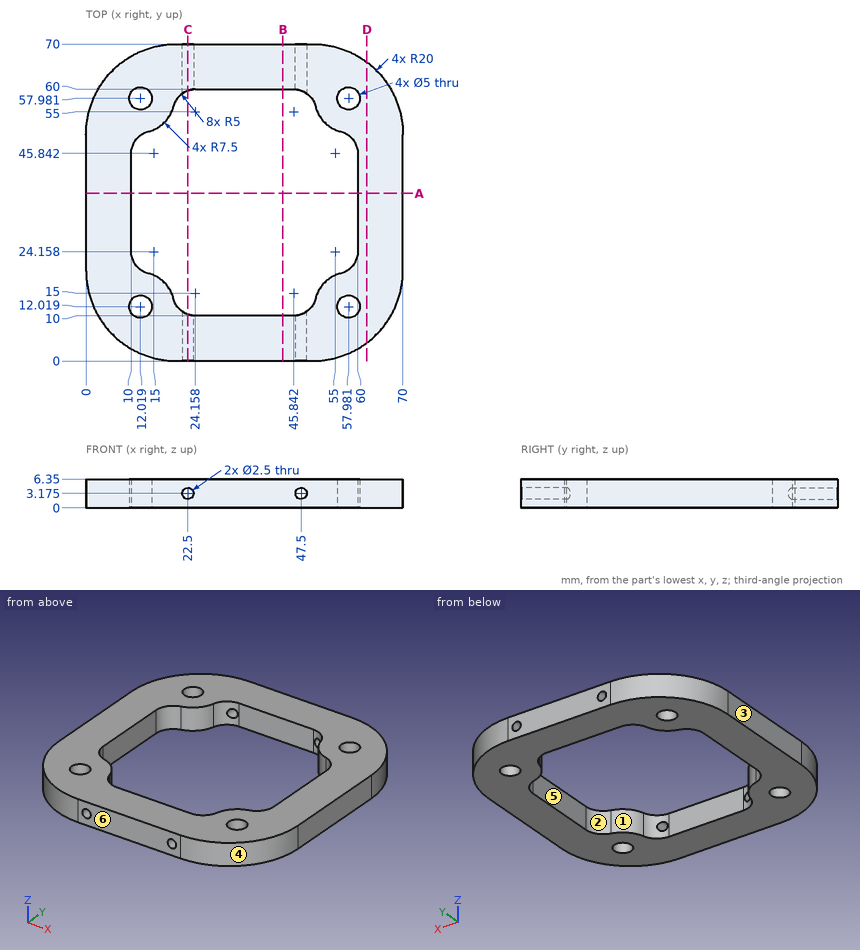
Answer from the drawing. Dimensions are ordinates in mm from the lowest x, y and z of the part. A direction names the side the tool comes from. Give positions to 0.01 mm unless a question says otherwise; leave off trailing zeros. Write each loop counter-clockwise with the first axis right and the second up, starting at its lowest first coordinate (ties: lowest second). Pieces come first, ordered by that corner, then holes. Notation, with made-up numbers: (-28, 40) - (16, 40) arc R32 cw to (16, 73) - close; hole circle Ø9 at (34, 36). An arc over 180 degrees is marked (long way). Answer in a Markdown table with one row per item. Add a question column.
Item 1: A tool of negligible diameter and unlimited length cuts with its end or side. For the marked faces 5 and 6, from which of +Z, -Z, +X, -X, +Y, -Y can it reach the whole face along a straight path? Write none if from no direction.
Item 2: Section A-A, the plane y = 37 is taken. Write down the section's boundary in (x, z), and give its area (3 significant figures).
Item 3: Determine the mould class of the marked faces 1, 2, 3 and 4 for opening direction Y: pulls with the +Y half, pulls with the -Y half, needs draft (parallel to the pull), parting line crosses it, or undercut.
Item 4: Flat-ended cylindrical pins translate along their axes: P1, Ø3, axis at y = 10, z = 5.5, coming from the -X side; P2, Ø1, axis at y = 56.5, z = 2.5, coming from the +X side. Find the tip coordinate at first contact, or state that the pin passes through.
Item 5: Section D-D, the plane x = 62 is taken. Write down the section's boundary in (y, z).
Item 6: Find the intervals of material crossed by L1, parallel to X at y = 28.5, z = 2.25; L2, parallel to Y at x = 10.5, z = 3 (1 decimal), in increasing order.
Item 7: Section C-C, the plane x = 22.5 is taken. Count the separate pieces of the cut face and the enclosed holes in it.
Recorded:
| question | item | result |
|---|---|---|
| 1 | face 5 | +Z, -Z |
| 1 | face 6 | +Z, -Z, +X, -X, -Y |
| 2 | outline | (0, 0) - (10, 0) - (10, 6.35) - (0, 6.35) - close; (60, 0) - (70, 0) - (70, 6.35) - (60, 6.35) - close |
| 2 | area | 127 mm2 |
| 3 | face 1 | undercut |
| 3 | face 2 | undercut |
| 3 | face 3 | needs draft |
| 3 | face 4 | pulls with the -Y half |
| 4 | P1 | stops at x = 1.9 |
| 4 | P2 | stops at x = 69.08 |
| 5 | outline | (4, 0) - (66, 0) - (66, 6.35) - (4, 6.35) - close |
| 6 | L1 | x = 0 to 10, 60 to 70 |
| 6 | L2 | y = 2.4 to 10, 14 to 22, 48 to 56, 60 to 67.6 |
| 7 | separate pieces | 4 |
| 7 | enclosed holes | 0 |
